Could you check a few things on this model? Use its own coordinates, in mm. A direction names the side the tool comes from. Round coordinates to 2 decimals unless told otherwise and drop trailing zeros. Loops run counter-clockwise (first coordinate to the right, second up) from the corner with the lowest first, then second, coordinate; pieces in that order, holes last. Notation, with made-up numbers: (-20, 75) -> (-12, 75) arc R24 cw to (-12, 89) -> close; hole circle Ø10 at (-14, -5.75). An arc over 180 degrees is marked (long way). Write each question's results on one line, items separated by ' | '. Start each with the question number.
1) Imagine slicing it at C-C, the plane x = -50. List the corners of the cut face in (y, z) for me.
2) If I drill on probe 1 along X at (y, z) = (5.25, 4.05); probe 2 along X at (y, z) = (4, 0.4); probe 3 along X at (y, z) = (-2, 0.25), over which ranges is the centre line in solid material (lowest first)?
3) We'd pull the mould along X, two halves only. Please class faces 4 (the flat face through (-62.6, 1, 2)), 5 (the flat face through (-0.609, 0, 3)), 6 (the flat face through (-31, 5.398, 2)), 7 (the flat face through (-61, -4.202, 2)): pulls with the +X half, pulls with the -X half, needs draft (parallel to the pull), parting line crosses it, or undercut.
4) Imagine slicing it at A-A, the plane z = 3.4. List the corners of the cut face in (x, y) for me.
5) For P1, Ø3, axis at x = 2, y = 0, coming from the +Z side; P2, Ø0.6, axis at x = 15, z = 0.5, coming from the -Y side; P3, Ø1.4, axis at x = -1.5, y = 0, coming from the +Z side; P4, Ø1.5, axis at x = -49, y = 4.5, coming from the -Z side, each with a flat end and sliding along its axis, tell me the tip position at first contact or that it passes through.
6) Imagine slicing it at B-B, the plane y = 1. List the corners of the cut face in (x, z) for me, plus the area to 3 significant figures.
7) Which directions (+Z, -Z, +X, -X, +Y, -Y) give clear straight access to the entire face, cutting with the end or side of a thin tool? Please do faces 1 (the flat face through (61, -4.202, 2)), 2 (the flat face through (-2, 0, 1.2)), 3 (the flat face through (-14, 6, 4.4)).
from build123d import *

# Parameters (mm, degrees)
F0_W     = 2.4
F0_H     = 9.6
F0_H_2   = 0.8
F0_W_2   = 1.2
F0_H_3   = 10
F0_W_3   = 1.6
F1_DEPTH = 4.4
F0_W_4   = 3.2
F0_H_4   = 1.6
F0_W_5   = 4.8
F2_DEPTH = 1.2
F3_DEPTH = 1


# Not quite as in the source:
# - ends of sketch curves that miss each other by under 0.0002 mm in the source are joined


with BuildPart() as f1:
    # F0 (on Top) → F1 (new body)
    with BuildSketch(Plane.XY):
        with Locations((-61.4, 0.5979961667)):
            Rectangle(F0_W, F0_H)
        with Locations((-61.4, 5.7979961667)):
            Rectangle(F0_W, F0_H_2)
        Polygon((-58.6, 5.3979961667), (-41.4000016928, 5.3979961667), (-38.2000016928, 5.3979961667), (-18.2000016928, 5.3979961667), (-13.4000016928, 5.3979961667), (-3.4000016928, 5.3979961667), (-0.6092149836, 5.3979961667), (0.5907850164, 5.3979961667), (3.3999983072, 5.3979961667), (13.4000016928, 5.3979961667), (18.2000016928, 5.3979961667), (38.2000016928, 5.3979961667), (41.4000016928, 5.3979961667), (58.6059018172, 5.3979961667), (58.6063936353, 6.1979961667), (-58.6, 6.1979961667), align=None)
        Polygon((62.5999775911, 6.1979961667), (60.1678602397, 6.1979961667), (60.1701559369, 5.3979961667), (62.5999775911, 5.3979961667), (62.5999775911, 5.7979961667), align=None)
        Polygon((62.5999775911, 5.3979961667), (60.1701559369, 5.3979961667), (60.1977043028, -4.2020038333), (62.6, -4.2020038333), align=None)
        with Locations((-0.0092149836, 0.3979961667)):
            Rectangle(F0_W_2, F0_H_3)
        with Locations((-59.4, 5.7979961667)):
            Rectangle(F0_W_3, F0_H_2)
        Polygon((60.1678602397, 6.1979961667), (58.6063936353, 6.1979961667), (58.6059018172, 5.3979961667), (60.1701559369, 5.3979961667), align=None)
    extrude(amount=F1_DEPTH)

    # F0 (on Top) → F2 (join)
    with BuildSketch(Plane.XY):
        with Locations((39.8000016928, 4.5979961667)):
            Rectangle(F0_W_4, F0_H_4)
        with Locations((15.8000016928, 4.9979961667)):
            Rectangle(F0_W_5, F0_H_2)
        with BuildLine():
            Line((3.3999983072, 5.3979961667), (0.5907850164, 5.3979961667))
            Line((0.5907850164, 5.3979961667), (0.5907850164, -4.6020038333))
            Line((0.5907850164, -4.6020038333), (1.7999983072, -4.6020038333))
            ThreePointArc((1.7999983072, -4.6020038333), (2.9313691571, -4.1333746832), (3.3999983072, -3.0020038333))
            Line((3.3999983072, -3.0020038333), (3.3999983072, 5.3979961667))
        make_face()
        with BuildLine():
            Line((-0.6092149836, 5.3979961667), (-3.4000016928, 5.3979961667))
            Line((-3.4000016928, 5.3979961667), (-3.4000016928, -3.0020038333))
            ThreePointArc((-3.4000016928, -3.0020038333), (-2.9313725427, -4.1333746832), (-1.8000016928, -4.6020038333))
            Line((-1.8000016928, -4.6020038333), (-0.6092149836, -4.6020038333))
            Line((-0.6092149836, -4.6020038333), (-0.6092149836, 5.3979961667))
        make_face()
        with Locations((-15.8000016928, 4.9979961667)):
            Rectangle(F0_W_5, F0_H_2)
        with Locations((-39.8000016928, 4.5979961667)):
            Rectangle(F0_W_4, F0_H_4)
    extrude(amount=F2_DEPTH)

    # F0 (on Top) → F3 (join)
    with BuildSketch(Plane.XY):
        with BuildLine():
            Line((-58.6, -3.4020038333), (-58.6, 5.3979961667))
            Line((-58.6, 5.3979961667), (-60.2, 5.3979961667))
            Line((-60.2, 5.3979961667), (-60.2, -4.2020038333))
            Line((-60.2, -4.2020038333), (-59.4, -4.2020038333))
            ThreePointArc((-59.4, -4.2020038333), (-58.8343145751, -3.9676892582), (-58.6, -3.4020038333))
        make_face()
        with BuildLine():
            Line((60.1701559369, 5.3979961667), (58.6059018172, 5.3979961667))
            Line((58.6059018172, 5.3979961667), (58.6004748691, -3.4295733769))
            ThreePointArc((58.6004748691, -3.4295733769), (58.8441470155, -3.9773540027), (59.3999996781, -4.2020038333))
            Line((59.3999996781, -4.2020038333), (60.1977043028, -4.2020038333))
            Line((60.1977043028, -4.2020038333), (60.1701559369, 5.3979961667))
        make_face()
    extrude(amount=F3_DEPTH)


solid = f1.part
Checked values:
1) outline: (5.4, 0) -> (6.2, 0) -> (6.2, 4.4) -> (5.4, 4.4) -> close
2) probe 1: -62.6 to -60.2, -0.61 to 0.59, 60.17 to 62.6 | probe 2: -62.6 to -58.6, -41.4 to -38.2, -3.4 to 3.4, 38.2 to 41.4, 58.61 to 62.6 | probe 3: -62.6 to -58.6, -3.4 to 3.4, 58.6 to 62.6
3) face 4: pulls with the -X half | face 5: undercut | face 6: undercut | face 7: needs draft
4) outline: (-62.6, -4.2) -> (-60.2, -4.2) -> (-60.2, 5.4) -> (-0.61, 5.4) -> (-0.61, -4.6) -> (0.59, -4.6) -> (0.59, 5.4) -> (60.17, 5.4) -> (60.2, -4.2) -> (62.6, -4.2) -> (62.6, 5.4) -> (62.6, 6.2) -> (-62.6, 6.2) -> close
5) P1: z = 4.4 | P2: y = 4.6 | P3: z = 1.2 | P4: through
6) outline: (-62.6, 0) -> (-58.6, 0) -> (-58.6, 1) -> (-60.2, 1) -> (-60.2, 4.4) -> (-62.6, 4.4) -> close; (-3.4, 0) -> (3.4, 0) -> (3.4, 1.2) -> (0.59, 1.2) -> (0.59, 4.4) -> (-0.61, 4.4) -> (-0.61, 1.2) -> (-3.4, 1.2) -> close; (58.6, 0) -> (62.6, 0) -> (62.6, 4.4) -> (60.18, 4.4) -> (60.18, 1) -> (58.6, 1) -> close | area: 36.4 mm^2
7) face 1: +Z, -Z, +X, -Y | face 2: +Z, -Y | face 3: +Z, +X, -X, +Y, -Y
